from build123d import *

# Parameters (mm, degrees)
SKETCH_1_R      = 1.5
SKETCH_1_R_2    = 1.25
SKETCH_1_R_3    = 14.1
EXTRUDE_1_DEPTH = 3


with BuildPart() as part:
    # 草图1 → 凸台-拉伸1 (new body)
    with BuildSketch(Plane(origin=(0, 0, 0), x_dir=(1, 0, 0), z_dir=(0, 1, 0))):
        Polygon((39.5, 13), (18.370549784, 12.991262473), (18.370549784, -13), (39.5, -13), (39.5, -28.031524747), (28.031524747, -39.5), (-22, -39.5), (-22, 30.5), (-22, 39.5), (28.031524747, 39.5), (39.5, 28.031524747), align=None)
        with Locations(Location((17.5, 35, 0), (0, 0, 270))):
            Circle(SKETCH_1_R, mode=Mode.SUBTRACT)
        with Locations(Location((22.337720199, 22.337720199, 0), (0, 0, 270))):
            Circle(SKETCH_1_R, mode=Mode.SUBTRACT)
        with Locations(Location((35, 17.5, 0), (0, 0, 270))):
            Circle(SKETCH_1_R, mode=Mode.SUBTRACT)
        with Locations(Location((17.5, -35, 0), (0, 0, 270))):
            Circle(SKETCH_1_R, mode=Mode.SUBTRACT)
        with Locations(Location((22.337720199, -22.337720199, 0), (0, 0, 270))):
            Circle(SKETCH_1_R, mode=Mode.SUBTRACT)
        with Locations(Location((35, -17.5, 0), (0, 0, 270))):
            Circle(SKETCH_1_R, mode=Mode.SUBTRACT)
        with Locations(Location((-14.1, 14.1, 0), (0, 0, 270))):
            Circle(SKETCH_1_R_2, mode=Mode.SUBTRACT)
        with Locations(Location((14.1, -14.1, 0), (0, 0, 270))):
            Circle(SKETCH_1_R_2, mode=Mode.SUBTRACT)
        with Locations(Location((0, 35, 0), (0, 0, 270))):
            Circle(SKETCH_1_R, mode=Mode.SUBTRACT)
        with Locations(Location((-17.5, 35, 0), (0, 0, 270))):
            Circle(SKETCH_1_R, mode=Mode.SUBTRACT)
        with Locations(Location((0, -35, 0), (0, 0, 90))):
            Circle(SKETCH_1_R, mode=Mode.SUBTRACT)
        with Locations(Location((-17.5, -35, 0), (0, 0, 90))):
            Circle(SKETCH_1_R, mode=Mode.SUBTRACT)
        with Locations(Location((14.1, 14.1, 0), (0, 0, 270))):
            Circle(SKETCH_1_R_2, mode=Mode.SUBTRACT)
        with Locations(Location((-14.1, -14.1, 0), (0, 0, 270))):
            Circle(SKETCH_1_R_2, mode=Mode.SUBTRACT)
        with Locations(Location((0, 0, 0), (0, 0, 270))):
            Circle(SKETCH_1_R_3, mode=Mode.SUBTRACT)
    extrude(amount=EXTRUDE_1_DEPTH)


solid = part.part
Can you work these out from the model? Positions are in its coordinate system, mm. A direction names the side the tool comes from. Give positions to 0.01 mm unless a question says otherwise; leave off trailing zeros. Order: outer loops, then holes, each group sorted by start corner. A loop starts at its lowest first (then second) coordinate and runs counter-clockwise, first axis right, second up. Notation, with made-up numbers: (84, -20) - (106, -20) arc R21 cw to (106, -14) - close; hole circle Ø3 at (33.25, 47.25). An arc over 180 degrees is marked (long way). Write each question's results on one line, items separated by ' | '.
1) Please list where these lines run through material, in increasing order: line 1 along Z through (x, y) = (25.5, 1.35); line 2 along X through (y, z) = (1.8, -17.5); line 3 along X through (y, z) = (1.8, -35). Write a range as [from, to].
Final values:
line 1: z = [-39.5, -12.99], [13, 39.5] | line 2: x = [-22, 33.5], [36.5, 39.5] | line 3: x = [-22, -19], [-16, -1.5], [1.5, 16], [19, 32.53]
2) I'm going to push flat-ended pins straight in: pin 1 Ø1.5 at (x, y) = (33.5, 1) entering from +Z; pin 2 Ø2.5 at (x, z) = (0, -35) entering from -Y. Where does each tip first touch, or does it pass through?
Final values:
pin 1: stops at z = 34.78 | pin 2: passes through
3) Suppose I cut it at B-B, the plane x = 0. Write out the boundary of the cut face in (y, z).
Final values:
outline: (0, -39.5) - (3, -39.5) - (3, -36.5) - (0, -36.5) - close; (0, -33.5) - (3, -33.5) - (3, -14.1) - (0, -14.1) - close; (0, 14.1) - (3, 14.1) - (3, 33.5) - (0, 33.5) - close; (0, 36.5) - (3, 36.5) - (3, 39.5) - (0, 39.5) - close
4) Suppose I cut it at D-D, the plane y = 0.8. Give the number of separate pieces and of enclosed holes in the cut face, then the cut area to 3 significant figures.
Final values:
separate pieces: 1 | enclosed holes: 15 | area: 3,460 mm^2
5) Suppose I cut it at A-A, the plane x = -17.5. Write out the boundary of the cut face in (y, z), then the cut area to 3 significant figures.
Final values:
outline: (0, -39.5) - (3, -39.5) - (3, -36.5) - (0, -36.5) - close; (0, -33.5) - (3, -33.5) - (3, 33.5) - (0, 33.5) - close; (0, 36.5) - (3, 36.5) - (3, 39.5) - (0, 39.5) - close | area: 219 mm^2
6) On a 3-axis mill with a long thin cutter (end or side, diameter ignored), from which of +Z, -Z, +X, -X, +Y, -Y can I reach the whole of each face in a straight line? I mean faces 5 (the face through (29, 1, 13)), 6 (the face through (20.873, 1.479, -22.663)). Say none if no direction works.
Final values:
face 5: +X, +Y, -Y | face 6: +Y, -Y
7) If we mould it in two halves opening along X, with no side actions, what happens to faces 1 (the face through (3, 1, -39.5)), 2 (the face through (13.34, 1.48, 13.11)), 3 (the face through (-22, 1, -1)), 4 (the face through (18.371, 1, 0))? For each: pulls with the +X half, pulls with the -X half, needs draft (parallel to the pull), parting line crosses it, or undercut.
Final values:
face 1: needs draft | face 2: undercut | face 3: pulls with the -X half | face 4: pulls with the +X half
8) Suppose I cut it at C-C, the plane z = 35. Write out the boundary of the cut face in (x, y), then the cut area to 3 significant figures.
Final values:
outline: (-22, 0) - (-19, 0) - (-19, 3) - (-22, 3) - close; (-16, 0) - (-1.5, 0) - (-1.5, 3) - (-16, 3) - close; (1.5, 0) - (16, 0) - (16, 3) - (1.5, 3) - close; (19, 0) - (32.53, 0) - (32.53, 3) - (19, 3) - close | area: 137 mm^2
